Could you check a few things on this model? Use its own coordinates, in mm. Face numbers are marked on the shaded views. A direction names the side the tool comes from. Round coordinates to 2 decimals unless told otherwise and drop trailing zeros. Loops run counter-clockwise (first coordinate to the right, second up) from the corner with the lowest first, then second, coordinate; pieces in that order, holes last. Notation, with made-up numbers: (-35.75, -15.5) -> (16.25, -15.5) arc R24 cw to (16.25, 13.5) -> close; hole circle Ø1 at (7.5, -36.5). An arc over 180 degrees is marked (long way). One line per item, written item: value.
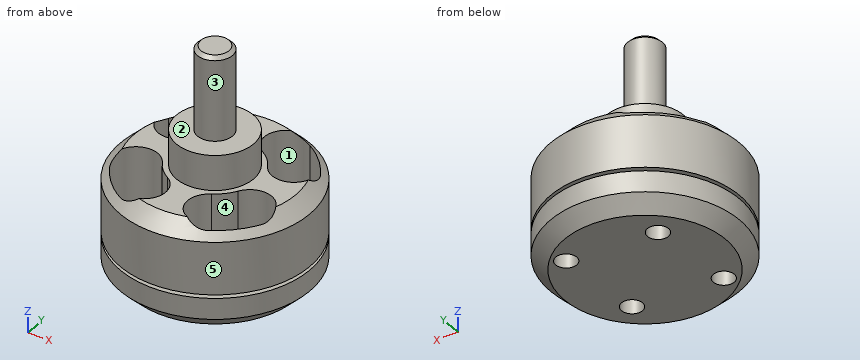
```python
from build123d import *

# Parameters (mm, degrees)
F2_SIZE  = 2
F3_SIZE  = 0.5
F6_DEPTH = 27.001
F7_R     = 1.5
F8_DEPTH = 4


with BuildPart() as f1:
    # F0 (on Front) → F1 (revolve)
    with BuildSketch(Plane.XZ):
        Polygon((0, 32), (0, 0), (13.5, 0), (13.5, 5), (2.5, 5), (2.5, 5.5), (13.5, 5.5), (13.5, 15), (5.5, 15), (5.5, 20), (2.5, 20), (2.5, 32), align=None)
    revolve(axis=Axis((0, 0, 16), (0, 0, -1)))

    # F2
    f2_edges = [f1.edges().sort_by_distance(p)[0] for p in [
        (-13.5, 0, 15),
        (-13.5, 0, 0),
    ]]
    chamfer(f2_edges, length=F2_SIZE)

    # F3
    f3_edges = [f1.edges().sort_by_distance(p)[0] for p in [
        (-2.5, 0, 32),
    ]]
    chamfer(f3_edges, length=F3_SIZE)

    # F5 (on offset) → F6 (cut, through all)
    with BuildSketch(Plane.XY.offset(5)):
        with BuildLine():
            ThreePointArc((5.412659, 3.125), (9.681488, 1.981171), (10.825318, 6.25))
            ThreePointArc((10.825318, 6.25), (8.838835, 8.838835), (6.25, 10.825318))
            ThreePointArc((6.25, 10.825318), (1.981171, 9.681488), (3.125, 5.412659))
            ThreePointArc((3.125, 5.412659), (4.419417, 4.419417), (5.412659, 3.125))
        make_face()
        with BuildLine():
            ThreePointArc((-3.125, 5.412659), (-1.981171, 9.681488), (-6.25, 10.825318))
            ThreePointArc((-6.25, 10.825318), (-8.838835, 8.838835), (-10.825318, 6.25))
            ThreePointArc((-10.825318, 6.25), (-9.681488, 1.981171), (-5.412659, 3.125))
            ThreePointArc((-5.412659, 3.125), (-4.419417, 4.419417), (-3.125, 5.412659))
        make_face()
        with BuildLine():
            ThreePointArc((-3.125, -5.412659), (-4.419417, -4.419417), (-5.412659, -3.125))
            ThreePointArc((-5.412659, -3.125), (-9.681488, -1.981171), (-10.825318, -6.25))
            ThreePointArc((-10.825318, -6.25), (-8.838835, -8.838835), (-6.25, -10.825318))
            ThreePointArc((-6.25, -10.825318), (-1.981171, -9.681488), (-3.125, -5.412659))
        make_face()
        with BuildLine():
            ThreePointArc((3.125, -5.412659), (1.981171, -9.681488), (6.25, -10.825318))
            ThreePointArc((6.25, -10.825318), (8.838835, -8.838835), (10.825318, -6.25))
            ThreePointArc((10.825318, -6.25), (9.681488, -1.981171), (5.412659, -3.125))
            ThreePointArc((5.412659, -3.125), (4.419417, -4.419417), (3.125, -5.412659))
        make_face()
    extrude(amount=F6_DEPTH, mode=Mode.SUBTRACT)

    # F7 (on Top) → F8 (cut)
    with BuildSketch(Plane.XY):
        with Locations((-5.656854, 5.656854)):
            Circle(F7_R)
        with Locations((6.717514, 6.717514)):
            Circle(F7_R)
        with Locations((5.656854, -5.656854)):
            Circle(F7_R)
        with Locations((-6.717514, -6.717514)):
            Circle(F7_R)
    extrude(amount=F8_DEPTH, mode=Mode.SUBTRACT)


solid = f1.part
```
Item 1: If we mould it in two halves opening along X, with no side actions, what happens to the marked faces 1, 2 and 3? For each: released by +X, released by -X, zero draft, split by the parting line, or undercut.
Output:
face 1: undercut
face 2: zero draft
face 3: split by the parting line
Item 2: I need wall thicknesses on line 1 (Y direction, x = 10.25, z = 9); line 2 (Y direction, x = 8.5, z = 9.5); line 3 (X direction, y = -5.5, z = 10). Which ranges of each line are inside material? Lowest first, please. Write a range as from..to.
Output:
line 1: y = -8.79..-7.15, -2.4..2.4, 7.15..8.79
line 2: y = -10.49..-9.17, -1.59..1.59, 9.17..10.49
line 3: x = -12.33..-11.14, -2.98..2.98, 11.14..12.33
Item 3: For the marked faces 4 and 5, which set-ups out of +Z, -Z, +X, -X, +Y, -Y let a thin tool reach every point of the face, with its end or its side?
Output:
face 4: +Z
face 5: +Z, -Z
Item 4: If we section it at B-B on y = 0: List the corners of the cut face in (x, z) for me, plus the area to 3 significant figures.
Output:
outline: (-13.5, 2) -> (-11.5, 0) -> (11.5, 0) -> (13.5, 2) -> (13.5, 5) -> (2.5, 5) -> (2.5, 5.5) -> (13.5, 5.5) -> (13.5, 13) -> (11.5, 15) -> (5.5, 15) -> (5.5, 20) -> (2.5, 20) -> (2.5, 31.5) -> (2, 32) -> (-2, 32) -> (-2.5, 31.5) -> (-2.5, 20) -> (-5.5, 20) -> (-5.5, 15) -> (-11.5, 15) -> (-13.5, 13) -> (-13.5, 5.5) -> (-2.5, 5.5) -> (-2.5, 5) -> (-13.5, 5) -> close
area: 501 mm²
Item 5: If we section it at D-D on z = 26.5: List the corners of the cut face in (x, y) for me, plus the area to 3 significant figures.
Output:
outline: circle Ø5 at (0, 0)
area: 19.6 mm²
Item 6: If we section it at A-A on z = 6: Count the separate pieces of the cut face and the enclosed holes in it, plus the area to 3 significant figures.
Output:
separate pieces: 1
enclosed holes: 4
area: 327 mm²
Item 7: Will these pins go through, and if not, where does the flat tip stop? pin 1 Ø0.9 at (x, y) = (6, 7) entering from -Z; pin 2 Ø5 at (y, z) = (-2, 20.5) entering from -X; pin 3 Ø1 at (x, y) = (-10, -2) entering from +Z.
Output:
pin 1: stops at z = 4
pin 2: stops at x = -5.5
pin 3: stops at z = 15
